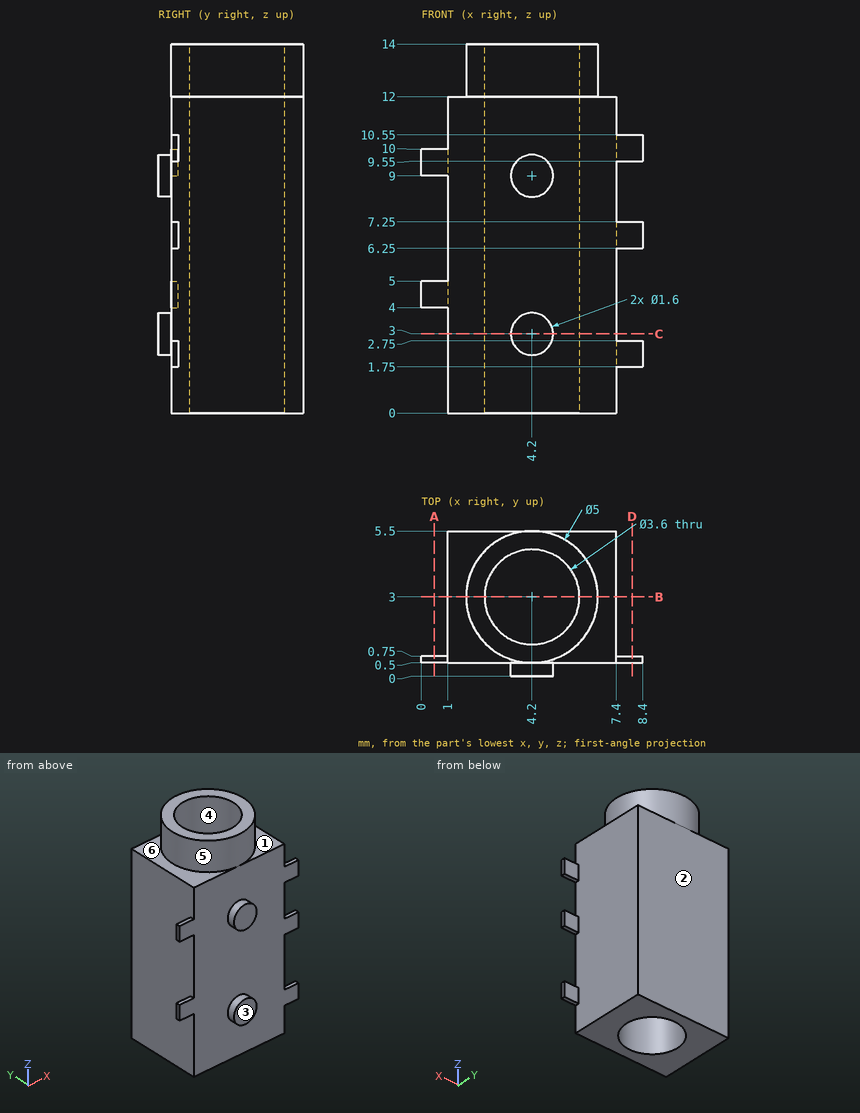
Geometry: see drawing. Coordinates: mm, zero at the bounding-box minimum. A direction names the side the tool comes from. Coordinates: 2 decimals unless noted, no trailing zeros. Loops run counter-clockwise (first coordinate to the right, second up) from the corner with the lowest first, then second, coordinate; pieces in that order, holes last.
(1) Section B-B on y = 3. Return the cut outline in (x, z), then the cut area to 3 significant figures.
(2) Set-up query: the marked faces 1 and 2. Return all of +Z, -Z, +X, -X, +Y, -Y with unobstructed straight access to the full face (end or side cutting, diameter ignored); none if empty.
(3) First-contact query: pin 1 Ø3 at (x, y) = (2, 3) entering from -Z; pin 2 Ø1.5 at (x, z) = (1, 7.5) entering from -Y; pin 3 Ø0.8 at (x, z) = (0.5, 9.5) entering from +Y. Flat tips, straight axial feed; report the tip coordinate or a pass-through.
(4) Pull-direction query (Y, two-part tool) for the marked faces 3, 4, 5 and 6; classes: released by +Y, released by -Y, zero draft, split by the parting line, or undercut.
(5) Material intervals for probe 1 along Y at (x, z) = (4.2, 6); probe 2 along Y at (x, z) = (4.2, 9); probe 3 along Y at (x, z) = (7.25, 9.25), sorted ascending.
(6) Section A-A on x = 0.5. Return the cut outline in (y, z).
(7) Section D-D on x = 8. Return the cut outline in (y, z).
(8) Section C-C on z = 3. Return the cut outline in (x, y).
Data:
1. outline: (1, 0) - (2.4, 0) - (2.4, 14) - (1.7, 14) - (1.7, 12) - (1, 12) - close; (6, 0) - (7.4, 0) - (7.4, 12) - (6.7, 12) - (6.7, 14) - (6, 14) - close
1. area: 36.4 mm2
2. face 1: +Z, +X
2. face 2: +Z, -Z, +X, -X, +Y
3. pin 1: stops at z = 0
3. pin 2: stops at y = 0.5
3. pin 3: stops at y = 0.75
4. face 3: released by -Y
4. face 4: undercut
4. face 5: split by the parting line
4. face 6: zero draft
5. probe 1: y = 0.5 to 1.2, 4.8 to 5.5
5. probe 2: y = 0 to 1.2, 4.8 to 5.5
5. probe 3: y = 0.5 to 5.5
6. outline: (0.5, 4) - (0.75, 4) - (0.75, 5) - (0.5, 5) - close; (0.5, 9) - (0.75, 9) - (0.75, 10) - (0.5, 10) - close
7. outline: (0.5, 1.75) - (0.75, 1.75) - (0.75, 2.75) - (0.5, 2.75) - close; (0.5, 6.25) - (0.75, 6.25) - (0.75, 7.25) - (0.5, 7.25) - close; (0.5, 9.55) - (0.75, 9.55) - (0.75, 10.55) - (0.5, 10.55) - close
8. outline: (1, 0.5) - (3.4, 0.5) - (3.4, 0) - (5, 0) - (5, 0.5) - (7.4, 0.5) - (7.4, 5.5) - (1, 5.5) - close; hole circle Ø3.6 at (4.2, 3)
